For this review, use the dimensioned drawing (mm, ordinates from the lowest corner) and the shaded views. A direction names the side the tool comes from. Coordinates: 2 decimals unless noted, no trailing zeros. Order: outer loops, then holes, each group sorted by start corner. A loop starts at its lowest first (then second) coordinate and runs counter-clockwise, first axis right, second up. Notation, with made-up numbers: (46.25, 45.25) -> (55.25, 45.25) arc R27 ccw to (55.25, 73.25) -> close; hole circle Ø4 at (58, -4). An arc over 180 degrees is marked (long way). Use one line per item in the form item = value. Start each with the question number.
(1) Insertion check: pin 1 Ø1 at (y, z) = (9.5, 28) entering from +X; pin 2 Ø1 at (x, y) = (28.5, 16.5) entering from +Z; pin 3 Ø4 at (x, z) = (21.5, 18.5) entering from +Y (1 decimal). Each pin has a flat end and moves straight along its axis. Give the tip position at first contact, or say it passes through.
(2) Mouldability with a two-part tool opening along X and no side actions: class the marked faces 1, 2 and 3 as +X half, -X half, draft (parallel to the pull), parting line (faces both ways), or undercut.
(3) Take a section at B-B (y = 4.5). State the section outline as (x, z) points, then the cut area to 3 significant figures.
(4) For the marked faces 4 and 5, list the 3-axis set-ups (+Z, -Z, +X, -X, +Y, -Y) from which the entire face can be reached by the end or side of a thin tool; tool diameter is ignored.
(5) Wall thickness on line 1 along Z through (x, y) = (19.05, 12.75); line 2 along Y through (x, z) = (11.5, 5); line 3 along Y through (x, z) = (14, 20.5) (1 decimal): over which ranges is each line inside the solid? List them lowest first.
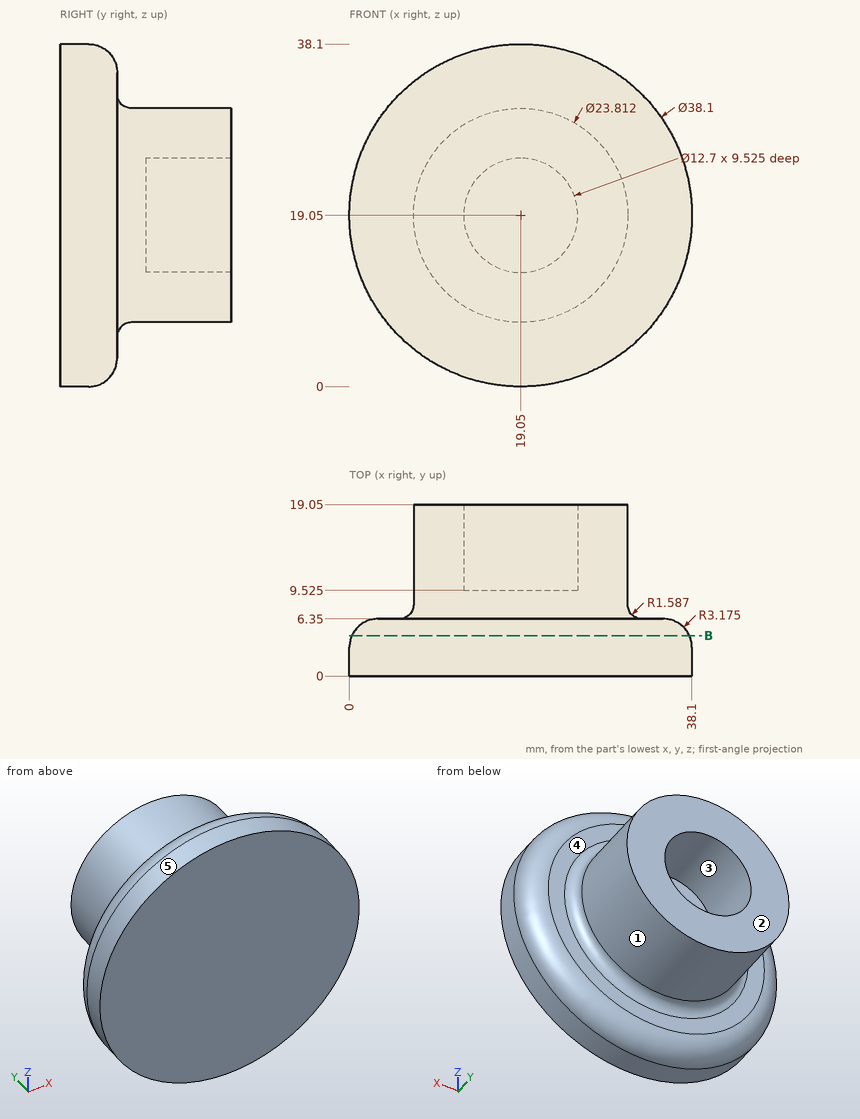
Findings:
q1.pin_1 = 27.44
q1.pin_2 = 26.9
q1.pin_3 = 9.5
q2.face_1 = parting line
q2.face_2 = draft
q2.face_3 = undercut
q3.outline = circle Ø37.52 at (19.05, 19.05)
q3.area = 1,110 mm²
q4.face_4 = +Y
q4.face_5 = +Y, -Y
q5.line_1 = 7.14 to 12.7, 25.4 to 30.96
q5.line_2 = 0 to 6.35
q5.line_3 = 0 to 9.5
